Work out the finished part from the listing and answer in its coordinate system (mm). A direction names the side the tool comes from. Give positions to 0.01 mm unless a question says otherwise; leave off trailing zeros. Loops run counter-clockwise (first coordinate to the right, second up) from the corner with the lowest first, then second, coordinate; pieces in that order, holes last. Notation, with made-up numbers: (-10, -22) - (24, -22) arc R10 cw to (24, -5) - close; hole circle Ø2 at (74, 76.25). An arc over 180 degrees is marked (long way). One line per item, written item: value.
Autodesk Inventor part; units mm, degrees
ref_plane "YZ Plane" through (0, 0, 0) normal (1, 0, 0) x (0, 1, 0)
ref_plane "XZ Plane" through (0, 0, 0) normal (0, 1, 0) x (-1, 0, 0)
ref_plane "XY Plane" through (0, 0, 0) normal (0, 0, 1) x (1, 0, 0)
sketch "スケッチ1" plane through (0, 0, 0) normal (0, 0, 1) x (1, 0, 0)
  line L0 (0, 0) -> (15, 0)
  line L1 (15, 0) -> (15, 15)
  line L2 (15, 15) -> (0, 15)
  line L3 (0, 15) -> (0, 0)
  dimension "d0" = 15
  dimension "d1" = 15
extrude "押し出し1" add sketch "スケッチ1" along normal blind 1.6
sketch "スケッチ2" plane through (0, 0, 1.6) normal (0, 0, 1) x (1, 0, 0)
  line L0 (1.25, 4) -> (13.75, 4)
  line L1 (13.75, 4) -> (13.75, 2.3)
  line L2 (13.75, 2.3) -> (1.25, 2.3)
  line L3 (1.25, 2.3) -> (1.25, 4)
  line L4 (0, 0) -> (15, 0)
  line L5 (15, 0) -> (15, 15)
  line L6 (15, 15) -> (0, 15)
  line L7 (0, 15) -> (0, 0)
  line L8 (0, 0) -> (15, 0)
  line L9 (0, 15) -> (0, 0)
  line L10 (0, 7.5) -> (2.3188, 7.5)
  line L11 (1.25, 11) -> (13.75, 11)
  line L12 (13.75, 11) -> (13.75, 12.7)
  line L13 (13.75, 12.7) -> (1.25, 12.7)
  line L14 (1.25, 12.7) -> (1.25, 11)
  line L15 (7.5, 2.3) -> (7.5, 0)
  point P0 (7.5, 13.5879)
  dimension "d4" = 12.5
  dimension "d5" = 1.7
  dimension "d6" = 7
extrude "押し出し2" cut sketch "スケッチ2" against normal through all contours L0 L1 L2 L3 | L14 L13 L12 L11
properties part number "USBブリッジ基板1"
1. For faces 4 (the flat face through (7, 8, 1.6)), 5 (the flat face through (13.75, 3, 1)), determine the directions among +Z, -Z, +X, -X, +Y, -Y from which every point of the face is accessible in a straight line to the end or side of a thin tool.
Output:
face 4: +Z, +X, -X, +Y, -Y
face 5: +Z, -Z
2. Section B-B (x = 9) is taken. Write down the section's boundary in (y, z).
Output:
outline: (0, 0) - (2.3, 0) - (2.3, 1.6) - (0, 1.6) - close; (4, 0) - (11, 0) - (11, 1.6) - (4, 1.6) - close; (12.7, 0) - (15, 0) - (15, 1.6) - (12.7, 1.6) - close
3. Find the intervals of material crossed by line 1 along Y through (x, z) = (8.5, 1); line 2 along X through (y, z) = (11.5, 0.45), in increasing order.
Output:
line 1: y = 0 to 2.3, 4 to 11, 12.7 to 15
line 2: x = 0 to 1.25, 13.75 to 15
4. Section C-C (z = 0.6) is taken. Write down the section's boundary in (x, y).
Output:
outline: (0, 0) - (15, 0) - (15, 15) - (0, 15) - close; hole (1.25, 2.3) - (13.75, 2.3) - (13.75, 4) - (1.25, 4) - close; hole (1.25, 11) - (13.75, 11) - (13.75, 12.7) - (1.25, 12.7) - close
5. The mould has two halves that part along Y. Classify faces 1 (the flat face through (8, 15, 1)), 2 (the flat face through (7, 0, 1)), 3 (the flat face through (13.75, 12, 1)): released by +Y, released by -Y, zero draft, split by the parting line, or undercut.
Output:
face 1: released by +Y
face 2: released by -Y
face 3: undercut
6. Section A-A (y = 2.5) is taken. Write down the section's boundary in (x, z).
Output:
outline: (0, 0) - (1.25, 0) - (1.25, 1.6) - (0, 1.6) - close; (13.75, 0) - (15, 0) - (15, 1.6) - (13.75, 1.6) - close
